Part model, mm, in its own coordinate system. Round coordinates to 2 decimals unless told otherwise and drop trailing zeros. Write each loop counter-clockwise with the first axis right and the second up, starting at its lowest first coordinate (ties: lowest second). Pieces come first, ordered by that corner, then holes. Notation, with made-up numbers: M 88,59.25 L 104,59.25 A24 ccw 104,70.25 Z; hole C 51.25,24 d10. An arc over 180 degrees is marked long. Use one line per item in the form item = value. Start each with the question number.
Item 1: Probe L1, parallel to X at y = 17, z = 0.25; L2, parallel to Z at x = -0.75, y = -171.5. List the from-to ranges inside material, lowest first.
Item 2: Cut at C-C, the plane x = -3. Give the cut face in (y, z), then the cut area to 3 significant figures.
Item 3: Flat gauge pin, fed straight in: pin 1 Ø1.5 at (y, z) = (112, -1.5) entering from -X. Where does the tip first touch, or does it go through?
Item 4: Cut at A-A, the plane y = -154.5. Give the cut face in (x, z).
Item 5: Cut at B-B, the plane z = -3. Give the cut face in (x, y).
from build123d import *

# Parameters (mm, degrees)
CYLINDER_R          = 5
CYLINDER_DEPTH      = 394
CYLINDER_ROLL_ANGLE = 90


with BuildPart() as part:
    # Cylinder → Cylinder (new body)
    with BuildSketch(Plane.XY):
        Circle(CYLINDER_R)
    extrude(amount=CYLINDER_DEPTH)


with BuildPart() as part_1:
    # Cylinder roll: moved
    add(part.part.rotate(Axis((0, 0, 0), (1, 0, 0)), CYLINDER_ROLL_ANGLE))


with BuildPart() as part_2:
    # Cylinder placement: moved
    add(part_1.part.moved(Location((0, 197, 0))))


solid = part_2.part
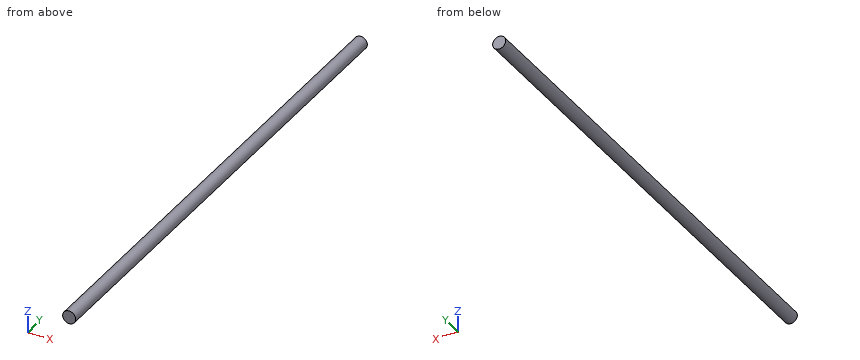
Model answer:
q1.L1 = -4.99 to 4.99
q1.L2 = -4.94 to 4.94
q2.outline = M -197,-4 L 197,-4 L 197,4 L -197,4 Z
q2.area = 3,150 mm²
q3.pin_1 = -4.94
q4.outline = C 0,0 d10
q5.outline = M -4,-197 L 4,-197 L 4,197 L -4,197 Z
